```python
from build123d import *
from OCP.BRepFilletAPI import BRepFilletAPI_MakeChamfer

# Parameters (mm, degrees)
SKETCH_1_W           = 7.11
SKETCH_1_H           = 6.22
EXTRUDE_1_DEPTH      = 2.62
CHAMFER_1_SIZE       = 1.2
CHAMFER_1_SIZE2      = 0.211592377
CHAMFER_2_SIZE       = 1
CHAMFER_2_SIZE2      = 0.176326981
SKETCH_3_W           = 1.589547356
SKETCH_3_H           = 0.4
CUT_EXTRUDE_1_DEPTH  = 8.628291093
EXTRUDE_2_DEPTH      = 1.6
EXTRUDE_2_DEPTH_BACK = 1.6
SKETCH_4_W           = 0.2
SKETCH_4_H           = 6.22
EXTRUDE_3_DEPTH      = 0.1


with BuildPart() as part:
    # 草图1 → 凸台-拉伸1 (new body)
    with BuildSketch(Plane(origin=(0, 0, 0), x_dir=(1, 0, 0), z_dir=(0, 1, 0))):
        Rectangle(SKETCH_1_W, SKETCH_1_H)
    extrude(amount=EXTRUDE_1_DEPTH)

    # 倒角1: one chamfer whose edges measure the first distance from different faces: ONE call of the kernel's chamfer builder (chamfer() names one face for all edges)
    chamfer_1_edges_1 = [part.edges().sort_by_distance(p)[0] for p in [
        (3.555, 2.62, 0),
    ]]
    chamfer_1_side_1 = [part.faces().sort_by_distance(p)[0] for p in [
        (3.555, 1.31, 0),
    ]]
    chamfer_1_edges_2 = [part.edges().sort_by_distance(p)[0] for p in [
        (-3.555, 2.62, 0),
    ]]
    chamfer_1_side_2 = [part.faces().sort_by_distance(p)[0] for p in [
        (-3.555, 1.31, 0),
    ]]
    chamfer_1 = BRepFilletAPI_MakeChamfer(part.part.solid().wrapped)
    for e in chamfer_1_edges_1:
        chamfer_1.Add(CHAMFER_1_SIZE, CHAMFER_1_SIZE2, e.wrapped, chamfer_1_side_1[0].wrapped)  # the first distance lies on this face
    for e in chamfer_1_edges_2:
        chamfer_1.Add(CHAMFER_1_SIZE, CHAMFER_1_SIZE2, e.wrapped, chamfer_1_side_2[0].wrapped)  # the first distance lies on this face
    add(Compound.cast(chamfer_1.Shape()), mode=Mode.REPLACE)

    # 倒角2: one chamfer whose edges measure the first distance from different faces: ONE call of the kernel's chamfer builder (chamfer() names one face for all edges)
    chamfer_2_edges_1 = [part.edges().sort_by_distance(p)[0] for p in [
        (3.555, 0, 0),
    ]]
    chamfer_2_side_1 = [part.faces().sort_by_distance(p)[0] for p in [
        (3.555, 0.71, 0),
    ]]
    chamfer_2_edges_2 = [part.edges().sort_by_distance(p)[0] for p in [
        (-3.555, 0, 0),
    ]]
    chamfer_2_side_2 = [part.faces().sort_by_distance(p)[0] for p in [
        (-3.555, 0.71, 0),
    ]]
    chamfer_2 = BRepFilletAPI_MakeChamfer(part.part.solid().wrapped)
    for e in chamfer_2_edges_1:
        chamfer_2.Add(CHAMFER_2_SIZE, CHAMFER_2_SIZE2, e.wrapped, chamfer_2_side_1[0].wrapped)  # the first distance lies on this face
    for e in chamfer_2_edges_2:
        chamfer_2.Add(CHAMFER_2_SIZE, CHAMFER_2_SIZE2, e.wrapped, chamfer_2_side_2[0].wrapped)  # the first distance lies on this face
    add(Compound.cast(chamfer_2.Shape()), mode=Mode.REPLACE)

    # 草图3 → 切除-拉伸1 (cut, through all)
    with BuildSketch(Plane.XY.offset(3.11)):
        with Locations((-3.34769153, 0.2)):
            Rectangle(SKETCH_3_W, SKETCH_3_H)
        with Locations((3.34769153, 0.2)):
            Rectangle(SKETCH_3_W, SKETCH_3_H)
    extrude(amount=-CUT_EXTRUDE_1_DEPTH, mode=Mode.SUBTRACT)

    # 草图2 → 凸台-拉伸2 (add, two sides: drawn at the far end of the back side and taken through both)
    with BuildSketch(Plane.XY.offset(-EXTRUDE_2_DEPTH_BACK)):
        with BuildLine():
            Line((3.311187824, 0.990859164), (3.311187824, 1.490859164))
            Line((3.311187824, 1.490859164), (3.922104584, 1.490859164))
            ThreePointArc((3.922104584, 1.490859164), (4.063525941, 1.43228052), (4.122104584, 1.290859164))
            Line((4.122104584, 1.290859164), (4.122104584, 0.297))
            ThreePointArc((4.122104584, 0.297), (3.975657975, -0.056553391), (3.622104584, -0.203))
            Line((3.622104584, -0.203), (2.711617897, -0.203))
            Line((2.711617897, -0.203), (2.711617897, 0.297))
            Line((2.711617897, 0.297), (3.422104584, 0.297))
            ThreePointArc((3.422104584, 0.297), (3.563525941, 0.355578644), (3.622104584, 0.497))
            Line((3.622104584, 0.497), (3.622104584, 0.790859164))
            ThreePointArc((3.622104584, 0.790859164), (3.563525941, 0.93228052), (3.422104584, 0.990859164))
            Line((3.422104584, 0.990859164), (3.311187824, 0.990859164))
        make_face()
        with BuildLine():
            Line((-3.311187824, 0.990859164), (-3.422104584, 0.990859164))
            ThreePointArc((-3.422104584, 0.990859164), (-3.563525941, 0.93228052), (-3.622104584, 0.790859164))
            Line((-3.622104584, 0.790859164), (-3.622104584, 0.497))
            ThreePointArc((-3.622104584, 0.497), (-3.563525941, 0.355578644), (-3.422104584, 0.297))
            Line((-3.422104584, 0.297), (-2.711617897, 0.297))
            Line((-2.711617897, 0.297), (-2.711617897, -0.203))
            Line((-2.711617897, -0.203), (-3.622104584, -0.203))
            ThreePointArc((-3.622104584, -0.203), (-3.975657975, -0.056553391), (-4.122104584, 0.297))
            Line((-4.122104584, 0.297), (-4.122104584, 1.290859164))
            ThreePointArc((-4.122104584, 1.290859164), (-4.063525941, 1.43228052), (-3.922104584, 1.490859164))
            Line((-3.922104584, 1.490859164), (-3.311187824, 1.490859164))
            Line((-3.311187824, 1.490859164), (-3.311187824, 0.990859164))
        make_face()
    extrude(amount=EXTRUDE_2_DEPTH + EXTRUDE_2_DEPTH_BACK)

    # 草图4 → 凸台-拉伸3 (add)
    with BuildSketch(Plane(origin=(0, 2.62, 0), x_dir=(1, 0, 0), z_dir=(0, 1, 0))):
        with Locations((-2.796130455, 0)):
            Rectangle(SKETCH_4_W, SKETCH_4_H)
    extrude(amount=EXTRUDE_3_DEPTH)


solid = part.part
```
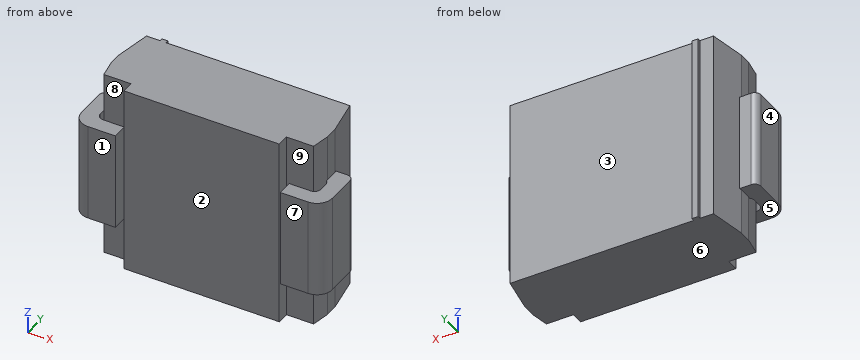
Input: part model. Units: mm. Frame: model coordinates. Face numbers are marked on the shaded views. A direction names the side the tool comes from. Coordinates: 2 decimals unless noted, no trailing zeros. Loops run counter-clockwise (first coordinate to the right, second up) from the corner with the lowest first, then second, coordinate; pieces in that order, holes last. Notation, with made-up numbers: (-24, 0.5) - (6, 0.5) arc R27 cw to (6, 17.5) - close; hole circle Ø11 at (33.5, 18.25). An arc over 180 degrees is marked (long way). Answer in a Markdown table with one row per item.
(1) Cut plane D-D on x = 0.25. Output: boundary loops of the cut face in (y, z).
Model answer:
| item | result |
|---|---|
| outline | (0, -3.11) - (2.62, -3.11) - (2.62, 3.11) - (0, 3.11) - close |
(2) Cut plane A-A on z = 2.5. Output: boundary loops of the cut face in (x, y) (3 decimals).
Model answer:
| item | result |
|---|---|
| outline | (-3.555, 1) - (-3.449, 0.4) - (-2.553, 0.4) - (-2.553, 0) - (2.553, 0) - (2.553, 0.4) - (3.449, 0.4) - (3.555, 1) - (3.555, 1.42) - (3.343, 2.62) - (-2.696, 2.62) - (-2.696, 2.72) - (-2.896, 2.72) - (-2.896, 2.62) - (-3.343, 2.62) - (-3.555, 1.42) - close |
(3) Pin query (flat end, axial travel): P1, Ø0.5, axis at x = -3, z = 0.5, coming from the +Y side; P2, Ø3, axis at x = 1, z = -0.5, coming from the +Y side. Return the tip coordinate at first contact, or that it passes through.
Model answer:
| item | result |
|---|---|
| P1 | stops at y = 2.72 |
| P2 | stops at y = 2.62 |
(4) Set-up query: the marked faces 1, 2, 3, 4 and 5. Return all of +Z, -Z, +X, -X, +Y, -Y with unobstructed straight access to the full face (end or side cutting, diameter ignored); none if empty.
Model answer:
| item | result |
|---|---|
| face 1 | +Z, -Z, +X, -X, -Y |
| face 2 | +Z, -Z, -Y |
| face 3 | +Z, -Z, +X, +Y |
| face 4 | +Z, -Z, -X, +Y, -Y |
| face 5 | -Z, -X, -Y |
(5) Material intervals for L1, parallel to Y at x = 0.5, z = 0.75; L2, parallel to Z at x = 3.75, y = 0.6; L3, parallel to Y at x = 4, z = 0, sorted ascending. Write a range as from..to.
Model answer:
| item | result |
|---|---|
| L1 | y = 0..2.62 |
| L2 | z = -1.6..1.6 |
| L3 | y = -0.03..1.48 |
(6) Cut plane B-B on y = 0.7. Output: boundary loops of the cut face in (x, z), plus the area to 3 significant figures.
Model answer:
| item | result |
|---|---|
| outline | (-4.12, -1.6) - (-3.62, -1.6) - (-3.62, 1.6) - (-4.12, 1.6) - close; (-3.5, -3.11) - (3.5, -3.11) - (3.5, 3.11) - (-3.5, 3.11) - close; (3.62, -1.6) - (4.12, -1.6) - (4.12, 1.6) - (3.62, 1.6) - close |
| area | 46.8 mm² |
(7) Cut plane C-C on y = 1.2. Output: boundary loops of the cut face in (x, z) (3 decimals).
Model answer:
| item | result |
|---|---|
| outline | (-4.122, -1.6) - (-3.555, -1.6) - (-3.555, -3.11) - (3.555, -3.11) - (3.555, -1.6) - (4.122, -1.6) - (4.122, 1.6) - (3.555, 1.6) - (3.555, 3.11) - (-3.555, 3.11) - (-3.555, 1.6) - (-4.122, 1.6) - close |
(8) Mould query, pull axis Y, two halves, no side actions, for the marked faces 6, 7, 8 and 9. Classes: pulls with the +Y half, pulls with the -Y half, needs draft (parallel to the pull), parting line crosses it, or undercut.
Model answer:
| item | result |
|---|---|
| face 6 | needs draft |
| face 7 | pulls with the -Y half |
| face 8 | undercut |
| face 9 | undercut |
